```python
from build123d import *

# Parameters (mm, degrees)
SKETCH1_W                      = 89
SKETCH1_H                      = 68
BASE_FLANGE2_DEPTH             = 1
EDGE_FLANGE1_STRIP_W           = 6
EDGE_FLANGE1_STRIP_H           = 1
EDGE_FLANGE1_STRIP_CUT_DEPTH   = 82.6
EDGE_FLANGE1_STRIP_2_W         = 6
EDGE_FLANGE1_STRIP_2_H         = 1
EDGE_FLANGE1_STRIP_CUT_2_DEPTH = 82.6
EDGE_FLANGE1_DEPTH             = 82.6
EDGE_FLANGE1_BEND_DEPTH        = 82.6
SKETCH16_W                     = 66.6
SKETCH16_H                     = 7
CUT_EXTRUDE1_DEPTH             = 138.553195479
FILLET1_R                      = 1
SKETCH17_R                     = 2
CUT_EXTRUDE2_DEPTH             = 138.553195479
M3_CLEARANCE_HOLE1_D           = 3.4
FILLET2_R                      = 2.5
SKETCH20_W                     = 8.5
SKETCH20_H                     = 68
BOSS_EXTRUDE1_DEPTH            = 1
FILLET3_R                      = 2.5


# Sheet-metal steps are written as plain solids
with BuildPart() as part:
    # Sketch1 → Base-Flange2 (new body)
    with BuildSketch(Plane(origin=(0, 0, 0), x_dir=(1, 0, 0), z_dir=(0, 1, 0))):
        Polygon((0, 0), (0, 82.6), (5, 82.6), (12.071067812, 89.671067812), (53.072, 89.671067812), (53.072, 79.921067812), (88.072, 79.921067812), (88.072, 89.671067812), (92.000932188, 89.671067812), (99.072, 82.6), (104.072, 82.6), (104.072, 0), (99.072, 0), (92.000932188, -7.071067812), (12.071067812, -7.071067812), (5, 0), align=None)
        with Locations((49.5, 41.5)):
            Rectangle(SKETCH1_W, SKETCH1_H, mode=Mode.SUBTRACT)
    extrude(amount=-BASE_FLANGE2_DEPTH)

    # Edge-Flange1 strip (across the edge) → Edge-Flange1 strip cut (cut)
    with BuildSketch(Plane(origin=(104.072, 0, 0), x_dir=(-1, 0, 0), z_dir=(0, 0, -1))):
        with Locations((-1, -0.5)):
            Rectangle(EDGE_FLANGE1_STRIP_W, EDGE_FLANGE1_STRIP_H)
    extrude(amount=EDGE_FLANGE1_STRIP_CUT_DEPTH, mode=Mode.SUBTRACT)

    # Edge-Flange1 strip 2 (across the edge) → Edge-Flange1 strip cut 2 (cut)
    with BuildSketch(Plane.XY.offset(-82.6)):
        with Locations((-1, -0.5)):
            Rectangle(EDGE_FLANGE1_STRIP_2_W, EDGE_FLANGE1_STRIP_2_H)
    extrude(amount=EDGE_FLANGE1_STRIP_CUT_2_DEPTH, mode=Mode.SUBTRACT)

    # Edge-Flange1 section (across the edge) → Edge-Flange1 (add)
    with BuildSketch(Plane(origin=(104.072, 0, 0), x_dir=(-1, 0, 0), z_dir=(0, 0, -1))):
        with BuildLine():
            Line((0, 1), (0, 7))
            Line((0, 7), (1, 7))
            Line((1, 7), (1, 1))
            ThreePointArc((1, 1), (1.292893219, 0.292893219), (2, 0))
            Line((2, 0), (2, -1))
            ThreePointArc((2, -1), (0.585786438, -0.414213562), (0, 1))
        make_face()
    extrude(amount=EDGE_FLANGE1_DEPTH)

    # Edge-Flange1 section 2 (across the edge) → Edge-Flange1 bend (add)
    with BuildSketch(Plane.XY.offset(-82.6)):
        with BuildLine():
            Line((0, 1), (0, 7))
            Line((0, 7), (1, 7))
            Line((1, 7), (1, 1))
            ThreePointArc((1, 1), (1.292893219, 0.292893219), (2, 0))
            Line((2, 0), (2, -1))
            ThreePointArc((2, -1), (0.585786438, -0.414213562), (0, 1))
        make_face()
    extrude(amount=EDGE_FLANGE1_BEND_DEPTH)

    # Sketch16 → Cut-Extrude1 (cut, through all)
    with BuildSketch(Plane(origin=(104.072, 0, 0), x_dir=(0, 0, -1), z_dir=(1, 0, 0))):
        with Locations((41.3, 4.5)):
            Rectangle(SKETCH16_W, SKETCH16_H)
    extrude(amount=-CUT_EXTRUDE1_DEPTH, mode=Mode.SUBTRACT)

    # Fillet1
    fillet1_edges = [part.edges().sort_by_distance(p)[0] for p in [
        (0.5, 7, -82.6),
        (0.5, 7, 0),
        (0.5, 7, -74.6),
        (0.5, 7, -8),
        (103.572, 7, -8),
        (103.572, 7, -74.6),
        (103.572, 7, 0),
        (103.572, 7, -82.6),
    ]]
    fillet(fillet1_edges, radius=FILLET1_R)

    # Sketch17 → Cut-Extrude2 (cut, through all)
    with BuildSketch(Plane(origin=(104.072, 0, 0), x_dir=(0, 0, -1), z_dir=(1, 0, 0))):
        with Locations(Location((4, 4, 0), (0, 0, 90))):
            Circle(SKETCH17_R)
        with Locations(Location((78.6, 4, 0), (0, 0, 90))):
            Circle(SKETCH17_R)
    extrude(amount=-CUT_EXTRUDE2_DEPTH, mode=Mode.SUBTRACT)

    # M3 Clearance Hole1 (through all)
    with Locations(Plane(origin=(0, -1, 0), x_dir=(-1, 0, 0), z_dir=(0, -1, 0))):
        with Locations((-93.299383015, 81.780067732), (-7.569381755, 77.970067732), (-7.569381755, 4.310067732), (-93.299383015, 1.770067732)):
            Hole(M3_CLEARANCE_HOLE1_D / 2)

    # Fillet2
    fillet2_edges = [part.edges().sort_by_distance(p)[0] for p in [
        (12.071067812, -0.5, -89.671067812),
        (53.072, -0.5, -89.671067812),
        (53.072, -0.5, -79.921067812),
        (88.072, -0.5, -79.921067812),
        (88.072, -0.5, -89.671067812),
        (92.000932188, -0.5, -89.671067812),
        (92.000932188, -0.5, 7.071067812),
        (12.071067812, -0.5, 7.071067812),
        (5, -0.5, -75.5),
        (94, -0.5, -75.5),
        (94, -0.5, -7.5),
        (5, -0.5, -7.5),
    ]]
    fillet(fillet2_edges, radius=FILLET2_R)

    # Sketch20 → Boss-Extrude1 (add)
    with BuildSketch(Plane.XZ.offset(1)):
        with Locations((29.25, -41.5)):
            Rectangle(SKETCH20_W, SKETCH20_H)
        with Locations((63.75, -41.5)):
            Rectangle(SKETCH20_W, SKETCH20_H)
    extrude(amount=-BOSS_EXTRUDE1_DEPTH)

    # Fillet3
    fillet3_edges = [part.edges().sort_by_distance(p)[0] for p in [
        (33.5, -0.5, -75.5),
        (25, -0.5, -75.5),
        (25, -0.5, -7.5),
        (33.5, -0.5, -7.5),
        (68, -0.5, -75.5),
        (59.5, -0.5, -75.5),
        (59.5, -0.5, -7.5),
        (68, -0.5, -7.5),
    ]]
    fillet(fillet3_edges, radius=FILLET3_R)


solid = part.part
```
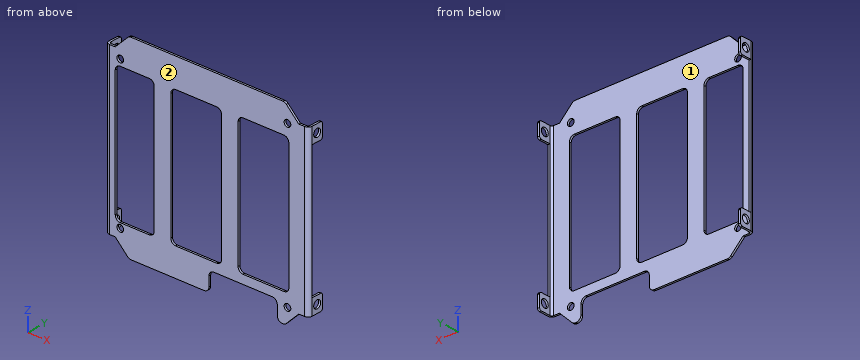
Source: CAD feature listing. Evaluate the final solid. Frame: model axes, mm. Face numbers are marked on the shaded views. Round coordinates to 2 decimals unless told otherwise and drop trailing zeros. Loops run counter-clockwise (first coordinate to the right, second up) from the corner with the lowest first, then second, coordinate; pieces in that order, holes last.
(1) Section query B-B (y = 4). Give the number of separate pieces and of enclosed holes in the cut face, and give its area (3 significant figures).
From the geometry:
separate pieces: 8
enclosed holes: 0
area: 16.0 mm2
(2) Section query A-A (x = 73.5). Output: boundary loops of the cut face in (y, z).
From the geometry:
outline: (-1, -79.92) - (0, -79.92) - (0, -75.5) - (-1, -75.5) - close; (-1, -7.5) - (0, -7.5) - (0, 7.07) - (-1, 7.07) - close
(3) Section query D-D (x = 40). Output: boundary loops of the cut face in (y, z).
From the geometry:
outline: (-1, -89.67) - (0, -89.67) - (0, -75.5) - (-1, -75.5) - close; (-1, -7.5) - (0, -7.5) - (0, 7.07) - (-1, 7.07) - close
(4) Contact query for flat-ended pins moving along their axis: pin 1 Ø0.5 at (y, z) = (-0.5, -49.5) entering from +X; pin 2 Ø1.1 at (y, z) = (-0.5, -84.5) entering from +X; pin 3 Ø3.5 at (y, z) = (4, -4) entering from +X; pin 4 Ø1.1 at (y, z) = (-0.5, -27.5) entering from -X. Output: stop coordinate, or through.
From the geometry:
pin 1: stops at x = 103.63
pin 2: stops at x = 97.72
pin 3: passes through
pin 4: stops at x = 0.24
(5) Pull-direction query (X, two-part tool) for the marked faces 1 and 2; classes: +X half, -X half, draft (parallel to the pull), parting line (faces both ways), or undercut.
From the geometry:
face 1: undercut
face 2: draft
(6) Material intervals for probe 1 along X at (y, z) = (4.75, -75); probe 2 along X at (y, z) = (-0.25, -43); probe 3 along X at (y, z) = (0.75, -53), sorted ascending.
From the geometry:
probe 1: x = 0 to 1, 103.07 to 104.07
probe 2: x = 0.44 to 5, 25 to 33.5, 59.5 to 68, 94 to 103.63
probe 3: x = 0.02 to 1.03, 103.04 to 104.06
(7) Section query C-C (z = -41.5). Output: boundary loops of the cut face in (x, y).
From the geometry:
outline: (0, 1) arc R2 ccw to (2, -1) - (5, -1) - (5, 0) - (2, 0) arc R1 cw to (1, 1) - close; (25, -1) - (33.5, -1) - (33.5, 0) - (25, 0) - close; (59.5, -1) - (68, -1) - (68, 0) - (59.5, 0) - close; (94, -1) - (102.07, -1) arc R2 ccw to (104.07, 1) - (103.07, 1) arc R1 cw to (102.07, 0) - (94, 0) - close
